Here's how the part is built. I have some questions about the finished solid (model axes, mm). A direction names the side the tool comes from. Give positions to 0.01 mm unless a question says otherwise; leave off trailing zeros. Order: outer loops, then holes, each group sorted by start corner. A loop starts at its lowest first (then second) coordinate and runs counter-clockwise, first axis right, second up. Notation, with made-up numbers: (6, 1) - (20, 1) arc R31 ccw to (20, 35) - close; hole circle Ø11 at (49, -30.5). An arc over 180 degrees is marked (long way). One line per question, with ' | ' between items.
from build123d import *

# Parameters (mm, degrees)
F1_DEPTH = 10.16
F2_R     = 2.8575
F2_R_2   = 2.54
F3_DEPTH = 25.4
F4_R     = 8.89


with BuildPart() as f1:
    # F0 (on Top) → F1 (new body)
    with BuildSketch(Plane.XY):
        with BuildLine():
            ThreePointArc((-21.838268, 2.290616), (-30.572093, -58.937184), (24.389732, -30.576631))
            ThreePointArc((24.389732, -30.576631), (18.146405, -10.688658), (1.656732, 2.062863))
            ThreePointArc((1.656732, 2.062863), (-10.070964, 4.219734), (-21.838268, 2.290616))
        make_face()
        with BuildLine():
            ThreePointArc((-21.838268, 2.290616), (-10.070964, 4.219734), (1.656732, 2.062863))
            Line((1.656732, 2.062863), (1.656732, 16.921369))
            Line((1.656732, 16.921369), (-21.838268, 16.921369))
            Line((-21.838268, 16.921369), (-21.838268, 2.290616))
        make_face()
    extrude(amount=F1_DEPTH)

    # F2 (on face) → F3 (cut)
    with BuildSketch(Plane.XY.offset(10.16)):
        with Locations((-21.838268, -15.159007)):
            Circle(F2_R)
        with Locations((-10.852768, -15.159007)):
            Circle(F2_R_2)
        with Locations((1.656732, -15.158281)):
            Circle(F2_R)
        with BuildLine():
            Line((2.609232, -51.658631), (2.609232, -36.418631))
            ThreePointArc((2.609232, -36.418631), (-10.090768, -23.718631), (-22.790768, -36.418631))
            Line((-22.790768, -36.418631), (-22.790768, -51.658631))
            ThreePointArc((-22.790768, -51.658631), (-10.090768, -64.358631), (2.609232, -51.658631))
        make_face()
    extrude(amount=-F3_DEPTH, mode=Mode.SUBTRACT)

    # F4
    f4_edges = [f1.edges().sort_by_distance(p)[0] for p in [
        (-21.838268, 16.921369, 5.08),
        (1.656732, 16.921369, 5.08),
    ]]
    fillet(f4_edges, radius=F4_R)


solid = f1.part
1) I want a section at B-B (y = -57.5). List the corners of the cut face in (x, z) for me, plus the area to 3 significant figures.
Model answer:
outline: (-32.45, 0) - (-21.37, 0) - (-21.37, 10.16) - (-32.45, 10.16) - close; (1.19, 0) - (11.64, 0) - (11.64, 10.16) - (1.19, 10.16) - close | area: 219 mm2
2) Thinking about a two-plate mould opening in Y: for faces 4 (the face through (1.657, 5, 5)), 5 (the face through (-9.81, -23.72, 5.15)), 6 (the face through (-1.02, 14.39, 5.15)), 7 (the face through (2.609, -44, 5)), which applies, +Y half, -Y half, draft (parallel to the pull), parting line (faces both ways), or undercut?
Model answer:
face 4: draft | face 5: undercut | face 6: +Y half | face 7: undercut
3) I want a section at C-C (z = 2.75). List the corners of the cut face in (x, y) for me (1 decimal), plus the area to 3 significant figures.
Model answer:
outline: (-21.8, 2.3) arc R34.8 ccw (long way) to (24.4, -30.6) arc R34.8 ccw to (1.7, 2.1) - (1.7, 8) arc R8.9 ccw to (-7.2, 16.9) - (-12.9, 16.9) arc R8.9 ccw to (-21.8, 8) - close; hole circle Ø5.7 at (-21.8, -15.2); hole (-22.8, -51.7) arc R12.7 ccw to (2.6, -51.7) - (2.6, -36.4) arc R12.7 ccw to (-22.8, -36.4) - close; hole circle Ø5.1 at (-10.9, -15.2); hole circle Ø5.7 at (1.7, -15.2) | area: 3,120 mm2
4) I'm going to push flat-ended pins straight in: P1, Ø3, axis at y = -47, z = 6, coming from the -X side; P2, Ø1, axis at y = -47.5, z = 8, coming from the -X side; P3, Ø5, axis at y = 5, z = 2.5, coming from the +X side. Where does each tip first touch, or does it pass through?
Model answer:
P1: stops at x = -41.84 | P2: stops at x = -41.09 | P3: stops at x = 1.66
5) Please list where these lines run through material, in increasing order: L1, parallel to X at y = -13, z = 7.5; L2, parallel to X at y = -31.5, z = 9.25; L3, parallel to Y at x = -18.5, z = 5.
Model answer:
L1: x = -40.44 to -23.71, -19.97 to -12.19, -9.51 to -0.22, 3.53 to 19.62 | L2: x = -45.19 to -21.8, 1.62 to 24.38 | L3: y = -64.42 to -61.18, -26.9 to 14.97
6) On a 3-axis mill with a long thin cutter (end or side, diameter ignored), from which of +Z, -Z, +X, -X, +Y, -Y can I reach the whole of each face in a straight line? I mean faces 1 (the face through (-10, 16.921, 5)), 2 (the face through (-22.791, -44, 5)), 3 (the face through (-21.838, 5, 5)). Say none if no direction works.
Model answer:
face 1: +Z, -Z, +X, -X, +Y | face 2: +Z, -Z | face 3: +Z, -Z, -X, +Y
7) I want a section at D-D (y = -19.5). List the corners of the cut face in (x, z) for me, plus the area to 3 significant figures.
Model answer:
outline: (-43.4, 0) - (22.58, 0) - (22.58, 10.16) - (-43.4, 10.16) - close | area: 670 mm2
8) I want a section at A-A (x = -16.5). List the corners of the cut face in (y, z) for me, plus the area to 3 significant figures.
Model answer:
outline: (-64.84, 0) - (-62.62, 0) - (-62.62, 10.16) - (-64.84, 10.16) - close; (-25.45, 0) - (16.18, 0) - (16.18, 10.16) - (-25.45, 10.16) - close | area: 446 mm2
